```python
from build123d import *

# Parameters (mm, degrees)
ESQUISSE1_R                        = 3.75
ESQUISSE1_R_2                      = 1.5
BOSS_EXTRU_1_DEPTH                 = 4
ENL_V_MAT_EXTRU_1_REACH            = 21.853
ESQUISSE2_R                        = 1.08
R_P_TITION_CIRCULAIRE1_COUNT       = 6
CONG_1_R                           = 11
ENL_V_MAT_EXTRU_2_REACH            = 21.853
CONG_2_R                           = 1
R_P_TITION_CIRCULAIRE2_COUNT       = 5
R_P_TITION_CIRCULAIRE2_ANGLE       = 240
CONG_2_OF_R_P_TITION_CIRCULAIRE2_R = 1


with BuildPart() as part:
    # Esquisse1 → Boss.-Extru.1 (new body)
    with BuildSketch(Plane.XY):
        with BuildLine():
            ThreePointArc((-9.34643428, 10.084972298), (6.875, -11.907849302), (-4.060625067, 13.13673567))
            ThreePointArc((-4.060625067, 13.13673567), (-7.596683666, 13.157842079), (-9.34643428, 10.084972298))
        make_face()
        Circle(ESQUISSE1_R, mode=Mode.SUBTRACT)
        with Locations((-5.846683666, 10.126753165)):
            Circle(ESQUISSE1_R_2, mode=Mode.SUBTRACT)
    extrude(amount=BOSS_EXTRU_1_DEPTH)

    # Esquisse2 → Enlèv. mat.-Extru.1 (cut, up to next)
    with BuildSketch(Plane.XY.offset(4), mode=Mode.PRIVATE) as enl_v_mat_extru_1_sk1:
        with Locations((0, 10.675)):
            Circle(ESQUISSE2_R)
    enl_v_mat_extru_1_tool1 = extrude(enl_v_mat_extru_1_sk1.sketch, amount=-ENL_V_MAT_EXTRU_1_REACH, mode=Mode.PRIVATE) & part.part
    enl_v_mat_extru_1 = enl_v_mat_extru_1_tool1.solids().sort_by_distance((0, 10.675, 4))[0]
    add(enl_v_mat_extru_1, mode=Mode.SUBTRACT)

    # Répétition circulaire1: Enlèv. mat.-Extru.1 ×6 about axis
    r_p_tition_circulaire1_axis = Axis((0, 0, 0), (0, 0, 1))
    for i in range(1, R_P_TITION_CIRCULAIRE1_COUNT):
        add(enl_v_mat_extru_1.rotate(r_p_tition_circulaire1_axis, i * 360 / R_P_TITION_CIRCULAIRE1_COUNT), mode=Mode.SUBTRACT)

    # Congé1
    cong_1_edges = [part.edges().sort_by_distance(p)[0] for p in [
        (-4.060625067, 13.13673567, 2),
        (-9.34643428, 10.084972298, 2),
    ]]
    fillet(cong_1_edges, radius=CONG_1_R)

    # Esquisse3 → Enlèv. mat.-Extru.2 (cut, up to next)
    with BuildSketch(Plane(origin=(0, 0, 0), x_dir=(-1, 0, 0), z_dir=(0, 0, -1)), mode=Mode.PRIVATE) as enl_v_mat_extru_2_sk1:
        with BuildLine():
            Line((-3.382940244, 10.729315696), (-1.879411247, 5.960730942))
            ThreePointArc((-1.879411247, 5.960730942), (-3.125, 5.412658774), (-4.222438798, 4.607983355))
            Line((-4.222438798, 4.607983355), (-7.600389836, 8.294370039))
            ThreePointArc((-7.600389836, 8.294370039), (-5.625, 9.742785793), (-3.382940244, 10.729315696))
        make_face()
    enl_v_mat_extru_2_tool1 = extrude(enl_v_mat_extru_2_sk1.sketch, amount=-ENL_V_MAT_EXTRU_2_REACH, mode=Mode.PRIVATE) & part.part
    enl_v_mat_extru_2 = enl_v_mat_extru_2_tool1.solids().sort_by_distance((4.458482, 7.722318, 0))[0]
    add(enl_v_mat_extru_2, mode=Mode.SUBTRACT)

    # Congé2
    cong_2_edges = [part.edges().sort_by_distance(p)[0] for p in [
        (7.600389836, 8.294370039, 2),
        (3.382940244, 10.729315696, 2),
        (1.879411247, 5.960730942, 2),
        (4.222438798, 4.607983355, 2),
    ]]
    fillet(cong_2_edges, radius=CONG_2_R)

    # Répétition circulaire2: Enlèv. mat.-Extru.2 ×5 about axis
    r_p_tition_circulaire2_axis = Axis((0, 0, 0), (0, 0, -1))
    for i in range(1, R_P_TITION_CIRCULAIRE2_COUNT):
        add(enl_v_mat_extru_2.rotate(r_p_tition_circulaire2_axis, i * R_P_TITION_CIRCULAIRE2_ANGLE / (R_P_TITION_CIRCULAIRE2_COUNT - 1)), mode=Mode.SUBTRACT)

    # Congé2 of Répétition circulaire2
    cong_2_of_r_p_tition_circulaire2_edges = [part.edges().sort_by_distance(p)[0] for p in [
        (10.98333008, -2.434945657, 2),
        (10.98333008, 2.434945657, 2),
        (6.101850044, 1.352747587, 2),
        (6.101850044, -1.352747587, 2),
        (3.382940244, -10.729315696, 2),
        (7.600389836, -8.294370039, 2),
        (4.222438798, -4.607983355, 2),
        (1.879411247, -5.960730942, 2),
        (-7.600389836, -8.294370039, 2),
        (-3.382940244, -10.729315696, 2),
        (-1.879411247, -5.960730942, 2),
        (-4.222438798, -4.607983355, 2),
        (-10.98333008, 2.434945657, 2),
        (-10.98333008, -2.434945657, 2),
        (-6.101850044, -1.352747587, 2),
        (-6.101850044, 1.352747587, 2),
    ]]
    fillet(cong_2_of_r_p_tition_circulaire2_edges, radius=CONG_2_OF_R_P_TITION_CIRCULAIRE2_R)


solid = part.part
```
Work out the finished part from the listing and answer in its coordinate system (mm). Coordinates: 2 decimals unless noted, no trailing zeros. Loops run counter-clockwise (first coordinate to the right, second up) from the corner with the lowest first, then second, coordinate; pieces in that order, holes last.
1) Section B-B (x = 0) is taken. Give the vertices of the cut face in (y, z) (3 decimals), plus the area to 3 significant figures.
Results:
outline: (-13.75, 0) - (-11.755, 0) - (-11.755, 4) - (-13.75, 4) - close; (-9.595, 0) - (-3.75, 0) - (-3.75, 4) - (-9.595, 4) - close; (3.75, 0) - (9.595, 0) - (9.595, 4) - (3.75, 4) - close; (11.755, 0) - (13.75, 0) - (13.75, 4) - (11.755, 4) - close
area: 62.7 mm2
2) Section C-C (x = 10.75) is taken. Give the vertices of the cut face in (y, z).
Results:
outline: (-8.57, 0) - (-2.05, 0) - (-2.05, 4) - (-8.57, 4) - close; (2.05, 0) - (8.57, 0) - (8.57, 4) - (2.05, 4) - close
3) Consider probe 1 along Y at (x, z) = (0, 2.15) (3 decimals); probe 2 along Y at (x, z) = (4.75, 1.1); probe 3 along X at (y, z) = (6.25, 2.25). Determine where each line is inside the solid, lowest interval first.
Results:
probe 1: y = -13.75 to -11.755, -9.595 to -3.75, 3.75 to 9.595, 11.755 to 13.75
probe 2: y = -12.9 to -10.2, -5.2 to 5.2, 10.2 to 12.9
probe 3: x = -12.25 to -9.82, -8.67 to 2.16, 5.73 to 8.67, 9.82 to 12.25
4) Section A-A (y = 0) is taken. Give the vertices of the cut face in (x, z), plus the area to 3 significant figures.
Results:
outline: (-13.75, 0) - (-11.25, 0) - (-11.25, 4) - (-13.75, 4) - close; (-6.25, 0) - (-3.75, 0) - (-3.75, 4) - (-6.25, 4) - close; (3.75, 0) - (6.25, 0) - (6.25, 4) - (3.75, 4) - close; (11.25, 0) - (13.75, 0) - (13.75, 4) - (11.25, 4) - close
area: 40.0 mm2
5) Section D-D (y = -11) is taken. Give the vertices of the cut face in (x, z), plus the area to 3 significant figures.
Results:
outline: (-8.25, 0) - (-1.03, 0) - (-1.03, 4) - (-8.25, 4) - close; (1.03, 0) - (8.25, 0) - (8.25, 4) - (1.03, 4) - close
area: 57.8 mm2
6) Flat-ended cylindrical pins translate along their axes: pin 1 (1 mm diameter, centred on x = -8.5, z = 2, fed in from -Y); pin 2 (2 mm diameter, centred on y = 5.5, z = 1.5, fed in from -X); pin 3 (1 mm diameter, centred on y = 7, z = 3.5, fed in from +X). Find the tip coordinate at first contact, or state that the pin passes through.
Results:
pin 1: stops at y = -11.18
pin 2: stops at x = -12.99
pin 3: stops at x = 12.12
